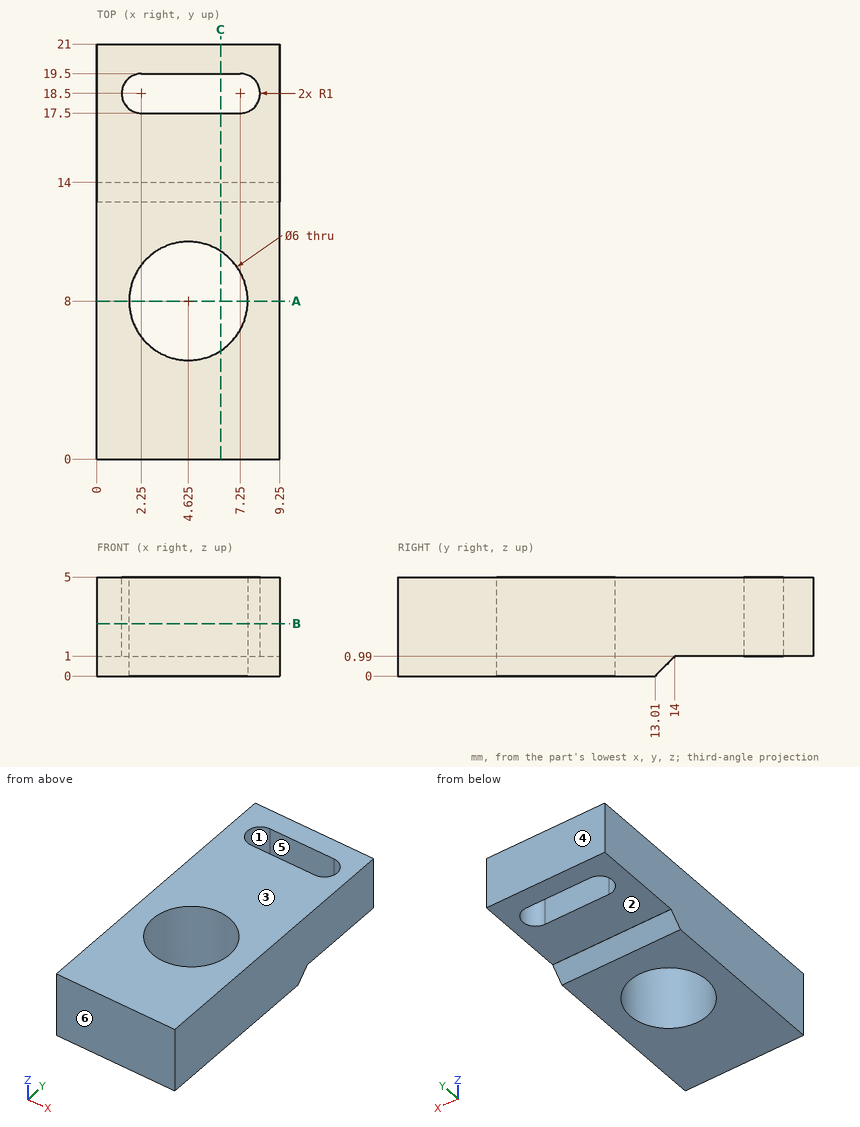
Could you check a few things on this drawing? It's one solid part, dimensions in mm from its lowest x, y, z. A direction names the side the tool comes from. Coordinates: 2 decimals unless noted, no trailing zeros. Order: outer loops, then holes, each group sorted by start corner. A loop starts at its lowest first (then second) coordinate and runs counter-clockwise, first axis right, second up. Notation, with made-up numbers: (56.25, 62.25) -> (93.25, 62.25) arc R24 ccw to (93.25, 82.25) -> close; hole circle Ø3 at (53.5, -26.5). An arc over 180 degrees is marked (long way). One line per item, written item: value. Start each with the question number.
1) Imagine slicing it at C-C on x = 6.25. Count the separate pieces of the cut face and the enclosed holes in it, plus the area to 3 significant figures.
2) Imagine slicing it at B-B on z = 2.65. List the corners of the cut face in (x, y) for me (3 decimals), plus the area to 3 significant figures.
3) Imagine slicing it at A-A on y = 8. List the corners of the cut face in (x, z) for me (3 decimals).
4) I'm going to push flat-ended pins straight in: pin 1 (1.5 mm diameter, centred on x = 6.5, y = 7.5, fed in from +Z) (3 decimals); pin 2 (3.5 mm diameter, centred on x = 4, y = 19, fed in from -Z). Where does each tip first touch, or does it pass through?
5) Which directions (+Z, -Z, +X, -X, +Y, -Y) give clear straight access to the entire face, cutting with the end or side of a thin tool? Please do the marked faces 1, 2 and 3.
6) If I drill on L1, parallel to Y at x = 4, z = 3.5; L2, parallel to Y at x = 5.75, z = 1.15; L3, parallel to X at y = 10.5, z = 3.65, over which ranges is the centre line in solid material (lowest first)? Write a range as [from, to].
7) We'd pull the mould along Y, two halves only. Please class the marked faces 4, 5 and 6: +Y half, -Y half, draft (parallel to the pull), parting line (faces both ways), or undercut.
Answer list:
1. separate pieces: 3
1. enclosed holes: 0
1. area: 64.3 mm2
2. outline: (0, 0) -> (9.25, 0) -> (9.25, 21) -> (0, 21) -> close; hole circle Ø6 at (4.625, 8); hole (2.25, 17.5) -> (7.25, 17.5) arc R1 ccw to (7.25, 19.5) -> (2.25, 19.5) arc R1 ccw to start
2. area: 153 mm2
3. outline: (0, 0) -> (1.625, 0) -> (1.625, 5) -> (0, 5) -> close; (7.625, 0) -> (9.25, 0) -> (9.25, 5) -> (7.625, 5) -> close
4. pin 1: passes through
4. pin 2: stops at z = 1
5. face 1: +Z, -Z
5. face 2: -Z, +X, -X, +Y
5. face 3: +Z, +X, -X, +Y, -Y
6. L1: y = [0, 5.07], [10.93, 17.5], [19.5, 21]
6. L2: y = [0, 5.22], [10.78, 17.5], [19.5, 21]
6. L3: x = [0, 2.97], [6.28, 9.25]
7. face 4: +Y half
7. face 5: undercut
7. face 6: -Y half
